Autodesk Inventor part; units mm, degrees
ref_plane "Start Plane" through (0, 0, -1.1225) normal (0, 0, 1) x (1, 0, 0)
ref_plane "End Plane" through (0, 0, 50) normal (0, 0, 1) x (1, 0, 0)
ref_plane "Work Plane4" through (1.5875, 0, -1.5875) normal (-0.7071, 0, -0.7071) x (-0.7071, 0, 0.7071)
ref_plane "Start Plane" through (0, 0, -1.1225) normal (0, 0, 1) x (1, 0, 0)
ref_plane "End Plane" through (0, 0, 50) normal (0, 0, 1) x (1, 0, 0)
sketch "Sketch" plane through (0, 0, 0) normal (0, 0, 1) x (1, 0, 0)
  circle A0 centre (0, 0) radius 1.5875
  dimension "d0" = 3.175
extrude "Body" add sketch "Sketch" along normal up to surface (51.1225 mm away) from surface at -1.1225
sketch "Sketch2" plane through (0, 0, 0) normal (0, 0, 1) x (1, 0, 0)
  line L0 (0, 0) -> (10, 0)
ref_plane "Work Plane3" through (0, 0, 0) normal (0, -1, 0) x (1, 0, 0)
sketch "Sketch3" plane through (0, 0, 0) normal (0, -1, 0) x (1, 0, 0)
  line L0 (-2, -1.1225) -> (12, -1.1225)
  line L1 (-2, 50) -> (12, 50)
  dimension "d7" = 51.1225
ref_plane "Work Plane4" through (1.5875, 0, -1.5875) normal (-0.7071, 0, -0.7071) x (-0.7071, 0, 0.7071)
split "Split1" plane through (1.5875, 0, -1.5875) removes the side toward (-0.7071, 0, -0.7071)
ref_plane "Work Plane5" through (0, 1.5875, -1.5875) normal (0, -0.7071, -0.7071) x (1, 0, 0)
split "Split2" plane through (0, 1.5875, -1.5875) removes the side toward (0, -0.7071, -0.7071)
equation "\"d0\" = Diam"
equation "\"d1\" = G_L"
equation "\"Diam\" = 3.175"
equation "\"G_L\" = d7"
equation "\"G_OFFSET_START\" = 1.12253"
equation "\"G_OFFSET_END\" = 0"
equation "\"d4\" = -G_OFFSET_START"
equation "\"d5\" = G_OFFSET_END + B_L"
equation "\"B_L\" = 50"
properties part number "ANSI/AISC Rolled Steel - 1/8-2,013, RB" material "Steel, Mild"
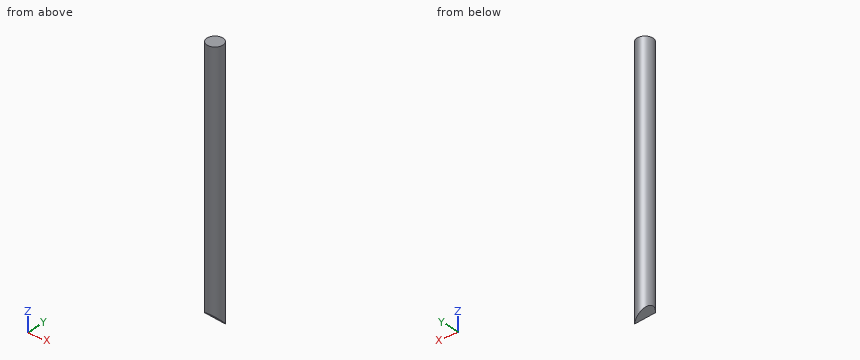
Can you work these out from the model? Positions are in its coordinate system, mm. Coordinates: 2 decimals unless noted, no trailing zeros. Order: outer loops, then holes, each group sorted by start corner. A loop starts at its lowest first (then second) coordinate and runs counter-clockwise, first axis right, second up. Notation, with made-up numbers: (-12, 48.25) - (10, 48.25) arc R23 ccw to (10, 61.25) - close; hole circle Ø10 at (9, 15). An arc over 180 degrees is marked (long way). Answer as a JSON object with one key per item and string values. Group by question number.
Q1. I need wall thicknesses on line 1 (Y direction, x = 0.15, z = 37); line 2 (Z direction, x = -0.9, y = -0.05); line 3 (Y direction, x = -1.2, z = 23). Which ranges of each line are inside material? Lowest first, please. Write a range as from..to.
Q2. Will this pin go through, and if not, where does the flat tip stop? P1, Ø1, axis at x = -0.5, z = 36, coming from the -Y side.
Q3. Imagine slicing it at C-C (z = 10). Please give me the cut outline in (x, y) (1 decimal).
Determined:
{
 "1": {"line 1": "y = -1.58..1.58", "line 2": "z = 0.9..50", "line 3": "y = -1.04..1.04"},
 "2": {"P1": "stops at y = -1.59"},
 "3": {"outline": "circle Ø3.2 at (0, 0)"}
}
